For this review, use the dimensioned drawing (mm, ordinates from the lowest corner) and the shaded views. A direction names the side the tool comes from. Coordinates: 2 decimals unless noted, no trailing zeros. Order: outer loops, then holes, each group sorted by start corner. A loop starts at its lowest first (then second) coordinate and runs counter-clockwise, first axis right, second up. Notation, with made-up numbers: (-6.75, 49.5) -> (21.25, 49.5) arc R22 ccw to (21.25, 56.5) -> close; hole circle Ø10 at (86.25, 34.5). An arc over 180 degrees is marked (long way). Return JSON: item names as keys, results as strings. Group by question number.
Item 1: Draft analysis for pull direction Z (two halves, no side actions). For the marked faces 3, 4 and 5, state which applies: +Z half, -Z half, draft (parallel to the pull), parting line (faces both ways), or undercut.
Item 2: Insertion check: pin 1 (7.5 mm diameter, centred on y = 13.5, z = 21.5, fed in from +X). The pin has a flat end and moves straight along its axis. Give the tip position at first contact, or say it passes through.
Item 3: For line 1 along Z through (x, y) = (82.55, 15.75); line 2 along Z through (x, y) = (19.05, 11); line 3 along Z through (x, y) = (61.5, 3.75), list the stretches that pass through material, from the lowest coordinate up.
Item 4: Machinability: for the marked faces 1 and 2, which of the approach directions +Z, -Z, +X, -X, +Y, -Y give a long, thin tool a straight path to every point of the face, cutting with its end or side? Answer none if there is none.
Item 5: Take a section at C-C (y = 10). Write out the cut boundary in (x, z).
Item 6: Take a section at A-A (x = 82.55). Write out the cut boundary in (y, z).
Item 7: Take a section at D-D (x = 19.05). Write out the cut boundary in (y, z), then the cut area to 3 significant figures.
Item 8: Take a section at B-B (z = 63.5). Write out the cut boundary in (x, y).
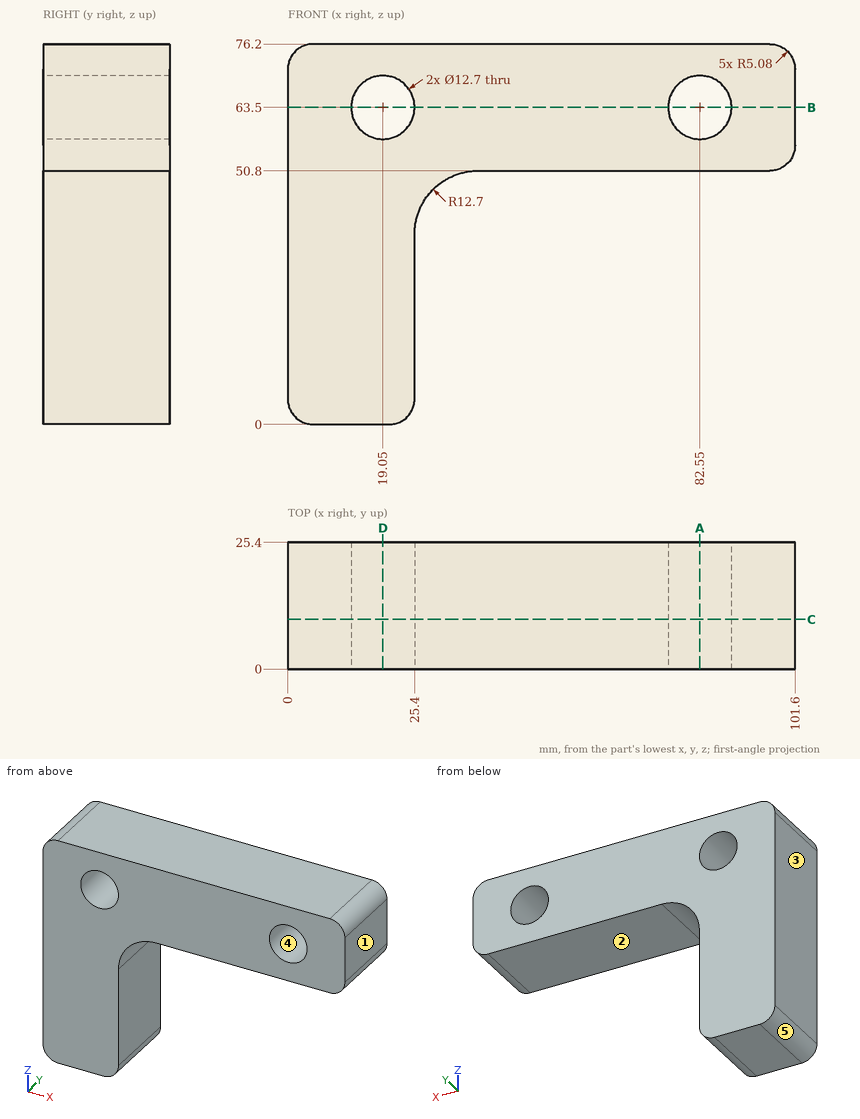
Findings below:
{
 "1": {"face 3": "draft", "face 4": "undercut", "face 5": "-Z half"},
 "2": {"pin 1": "stops at x = 25.4"},
 "3": {"line 1": "z = 50.8 to 57.15, 69.85 to 76.2", "line 2": "z = 0 to 57.15, 69.85 to 76.2", "line 3": "z = 50.8 to 76.2"},
 "4": {"face 1": "+Z, -Z, +X, +Y, -Y", "face 2": "-Z, +X, +Y, -Y"},
 "5": {"outline": "(0, 5.08) arc R5.08 ccw to (5.08, 0) -> (20.32, 0) arc R5.08 ccw to (25.4, 5.08) -> (25.4, 38.1) arc R12.7 cw to (38.1, 50.8) -> (96.52, 50.8) arc R5.08 ccw to (101.6, 55.88) -> (101.6, 71.12) arc R5.08 ccw to (96.52, 76.2) -> (5.08, 76.2) arc R5.08 ccw to (0, 71.12) -> close; hole circle Ø12.7 at (19.05, 63.5); hole circle Ø12.7 at (82.55, 63.5)"},
 "6": {"outline": "(0, 50.8) -> (25.4, 50.8) -> (25.4, 57.15) -> (0, 57.15) -> close; (0, 69.85) -> (25.4, 69.85) -> (25.4, 76.2) -> (0, 76.2) -> close"},
 "7": {"outline": "(0, 0) -> (25.4, 0) -> (25.4, 57.15) -> (0, 57.15) -> close; (0, 69.85) -> (25.4, 69.85) -> (25.4, 76.2) -> (0, 76.2) -> close", "area": "1,610 mm2"},
 "8": {"outline": "(0, 0) -> (12.7, 0) -> (12.7, 25.4) -> (0, 25.4) -> close; (25.4, 0) -> (76.2, 0) -> (76.2, 25.4) -> (25.4, 25.4) -> close; (88.9, 0) -> (101.6, 0) -> (101.6, 25.4) -> (88.9, 25.4) -> close"}
}
